```python
from build123d import *

# Parameters (mm, degrees)
F0_R      = 50
F1_DEPTH  = 6
F2_SIZE   = 5.99999
F4_DEPTH  = 57.5
F5_W      = 15
F5_H      = 28.75
F6_DEPTH  = 6
F7_W      = 154
F7_H      = 78
F8_DEPTH  = 1
F9_SIZE   = 9.99999
F10_R     = 2.2025754481
F11_DEPTH = 0.3
F12_DEPTH = 0.35
F13_R     = 2
F13_R_2   = 0.5
F14_DEPTH = 2


# Not quite as in the source:
# - a fillet or chamfer is up to 0.001 mm smaller than in the source, because OpenCascade refuses the exact size


with BuildPart() as f1:
    # F0 (on Front) → F1 (new body)
    with BuildSketch(Plane.XZ):
        with Locations((-39.6165661514, 33.0943278968)):
            Circle(F0_R)
    extrude(amount=F1_DEPTH)

    # F2 (size 6 in the source; OpenCascade refuses exactly that, so slightly less here)
    f2_edges = [f1.edges().sort_by_distance(p)[0] for p in [
        (-89.616566, -6, 33.094328),
    ]]
    chamfer(f2_edges, length=F2_SIZE)

    # F3 (on face) → F4 (join)
    with BuildSketch(Plane.XZ.offset(6)):
        Polygon((-54.6165661514, 28.0943278968), (-39.6165661514, 28.0943278968), (-24.6165661514, 28.0943278968), (-24.6165661514, 38.0943278968), (-39.6165661514, 38.0943278968), (-54.6165661514, 38.0943278968), align=None)
    extrude(amount=F4_DEPTH)

    # F5 (on face) → F6 (join)
    with BuildSketch(Plane(origin=(0, 0, 28.0943278968), x_dir=(1, 0, 0), z_dir=(0, 0, -1))):
        Polygon((-119.6165661514, 34.75), (-54.6165661514, 34.75), (-54.6165661514, 63.5), (-39.6165661514, 63.5), (-24.6165661514, 63.5), (-24.6165661514, 34.75), (40.3834338486, 34.75), (40.3834338486, 124.75), (-39.6165661514, 124.75), (-119.6165661514, 124.75), align=None)
        with Locations((-32.1165661514, 49.125)):
            Rectangle(F5_W, F5_H)
        with Locations((-47.1165661514, 49.125)):
            Rectangle(F5_W, F5_H)
    extrude(amount=F6_DEPTH)

    # F7 (on face) → F8 (cut)
    with BuildSketch(Plane(origin=(0, 0, 22.0943278968), x_dir=(1, 0, 0), z_dir=(0, 0, -1))):
        with Locations((-39.6165661514, 82.5612554252)):
            Rectangle(F7_W, F7_H)
    extrude(amount=-F8_DEPTH, mode=Mode.SUBTRACT)

    # F9 (size 10 in the source; OpenCascade refuses exactly that, so slightly less here)
    f9_edges = [f1.edges().sort_by_distance(p)[0] for p in [
        (-39.616566, -63.5, 38.094328),
    ]]
    chamfer(f9_edges, length=F9_SIZE)

    # F10 (on face) → F11 (join)
    with BuildSketch(Plane(origin=(0, 0, 22.0943278968), x_dir=(1, 0, 0), z_dir=(0, 0, -1))):
        with Locations((32.0070236921, 39.2166003585)):
            Circle(F10_R)
        with BuildLine():
            ThreePointArc((33.2229098133, 40.4324864797), (32.0070236921, 37.4970777156), (30.7911375709, 40.4324864797))
            ThreePointArc((30.7911375709, 40.4324864797), (31.1349833923, 40.4324864797), (31.1349833923, 40.0886406584))
            ThreePointArc((31.1349833923, 40.0886406584), (32.0070236921, 37.9833491395), (32.879063992, 40.0886406584))
            ThreePointArc((32.879063992, 40.0886406584), (32.879063992, 40.4324864797), (33.2229098133, 40.4324864797))
        make_face(mode=Mode.SUBTRACT)
        with BuildLine():
            ThreePointArc((32.2499889227, 39.2166003585), (32.0070236921, 38.9736351279), (31.7640584616, 39.2166003585))
            Line((31.7640584616, 39.2166003585), (31.7640584616, 40.6014584005))
            ThreePointArc((31.7640584616, 40.6014584005), (32.0070236921, 40.844423631), (32.2499889227, 40.6014584005))
            Line((32.2499889227, 40.6014584005), (32.2499889227, 39.2166003585))
        make_face(mode=Mode.SUBTRACT)
    extrude(amount=F11_DEPTH)

    # F12 (add): faces of the model
    f12_faces = [f1.faces().sort_by_distance(p)[0] for p in [
        (32.0070236921, -39.9090293795, 22.0943278968),
        (32.0070236921, -37.5427579145, 22.0943278968),
    ]]
    extrude(f12_faces, amount=F12_DEPTH)

    # F13 (on face) → F14 (cut)
    with BuildSketch(Plane.XY.offset(38.0943278968)):
        with Locations((-28.6587122828, -48.3524724841)):
            Circle(F13_R)
        with Locations((-28.6587122828, -48.3524724841)):
            Circle(F13_R_2, mode=Mode.SUBTRACT)
    extrude(amount=-F14_DEPTH, mode=Mode.SUBTRACT)


solid = f1.part
```
Here's how the part is built. I have some questions about the finished solid (model axes, mm). A direction names the side the tool comes from. Give positions to 0.01 mm unless a question says otherwise; leave off trailing zeros. Order: outer loops, then holes, each group sorted by start corner. A loop starts at its lowest first (then second) coordinate and runs counter-clockwise, first axis right, second up. Notation, with made-up numbers: (-26.75, 1.25) - (-19.75, 1.25) arc R19 ccw to (-19.75, 28.25) - close; hole circle Ø3 at (1, -30.5). An arc over 180 degrees is marked (long way). Answer as a JSON object with one key per item and string values. Group by question number.
Item 1: For P1, Ø2, axis at x = -28.5, y = -49, coming from the +Z side; P2, Ø12, axis at x = -59, y = -16, coming from the -Z side; P3, Ø8, axis at y = -33, z = 35.5, coming from the -X side; P4, Ø12, axis at x = 11, y = -15, coming from the +Z side (1 decimal), each with a flat end and sliding along its axis, tell me the tip position at first contact or that it passes through.
Item 2: If we section it at D-D on y = -57.5: Please give me the cut outline in (x, z), and give its area (3 significant figures).
Item 3: If we section it at B-B on y = -82.5: Please give me the cut outline in (x, z), and give its area (3 significant figures).
Item 4: If we mould it in two halves opening along X, with no side actions, what happens to faces 1 (the flat face through (-28, -49, 36.094)), 2 (the flat face through (-40, -20, 28.094)), 3 (the conical face through (-45.38, -5.71, 77.01))? For each: pulls with the +X half, pulls with the -X half, needs draft (parallel to the pull), parting line crosses it, or undercut.
Item 5: Please list where these lines run through material, in increasing order: probe 1 along Y at (x, z) = (-22, 35); probe 2 along Z at (x, y) = (25, -113.5); probe 3 along X at (y, z) = (-11, 30.5).
Item 6: If we section it at A-A on x = 27.5: Please give me the cut outline in (y, z).
Item 7: Which directions (+Z, -Z, +X, -X, +Y, -Y) give clear straight access to the entire face, cutting with the end or side of a thin tool? Please do faces 4 (the flat face through (-24.617, -34, 33)), 5 (the cylindrical face through (-27.74, -50.13, 37.11)), 6 (the flat face through (-39, -29, 38.094)), 7 (the flat face through (-41, -83, 23.094)).
Item 8: If we section it at C-C on y = -31: Please give me the cut outline in (x, z), and give its area (3 significant figures).
Result set:
{
 "1": {"P1": "z = 38.09", "P2": "z = 28.09", "P3": "x = -54.62", "P4": "through"},
 "2": {"outline": "(-119.62, 22.09) - (-116.62, 22.09) - (-116.62, 23.09) - (37.38, 23.09) - (37.38, 22.09) - (40.38, 22.09) - (40.38, 28.09) - (-24.62, 28.09) - (-24.62, 34.09) - (-54.62, 34.09) - (-54.62, 28.09) - (-119.62, 28.09) - close", "area": "986 mm²"},
 "3": {"outline": "(-119.62, 22.09) - (-116.62, 22.09) - (-116.62, 23.09) - (37.38, 23.09) - (37.38, 22.09) - (40.38, 22.09) - (40.38, 28.09) - (-119.62, 28.09) - close", "area": "806 mm²"},
 "4": {"face 1": "undercut", "face 2": "needs draft", "face 3": "parting line crosses it"},
 "5": {"probe 1": "-6 to 0", "probe 2": "23.09 to 28.09", "probe 3": "-54.62 to -24.62"},
 "6": {"outline": "(-124.75, 22.09) - (-121.56, 22.09) - (-121.56, 23.09) - (-43.56, 23.09) - (-43.56, 22.09) - (-34.75, 22.09) - (-34.75, 28.09) - (-124.75, 28.09) - close"},
 "7": {"face 4": "+Z, +X, -Y", "face 5": "+Z", "face 6": "+Z, +X, -X, -Y", "face 7": "-Z"},
 "8": {"outline": "(-54.62, 28.09) - (-24.62, 28.09) - (-24.62, 38.09) - (-54.62, 38.09) - close", "area": "300 mm²"}
}
